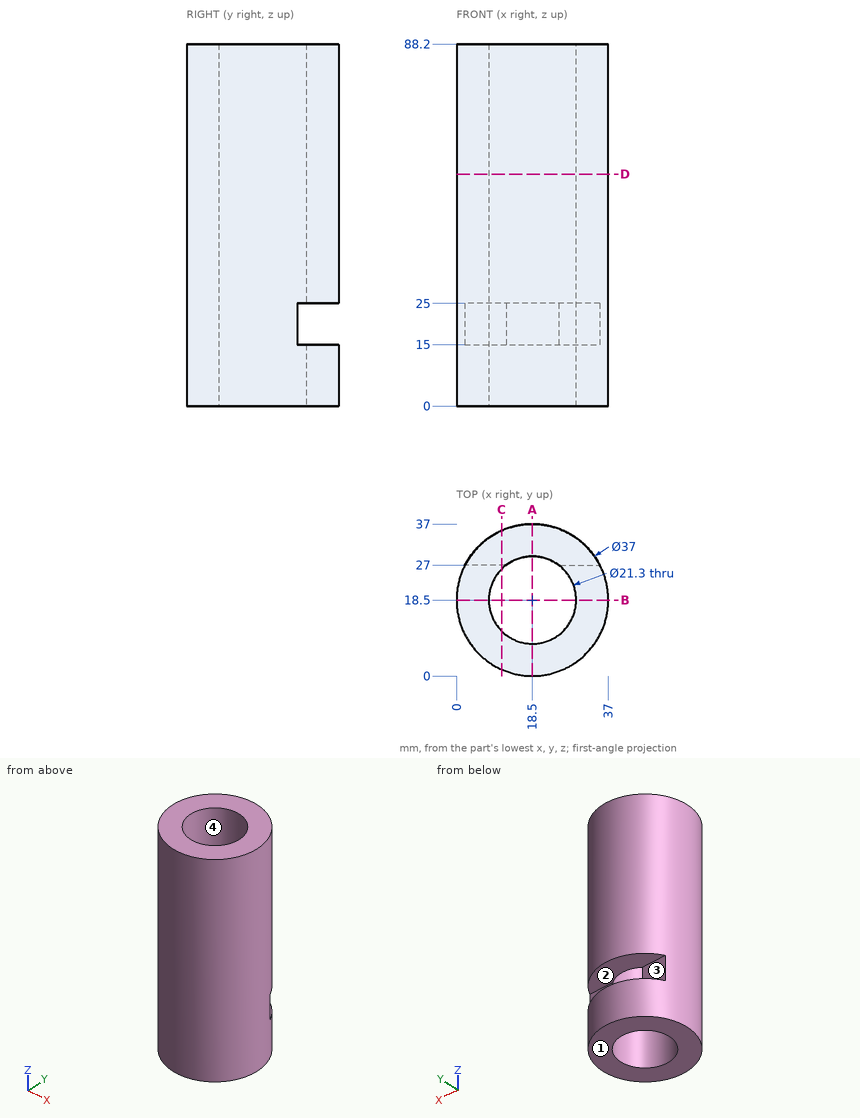
Answer from the drawing. Dimensions are ordinates in mm from the lowest x, y and z of the part. Give positions to 0.01 mm unless a question says otherwise; leave off trailing zeros. Order: outer loops, then holes, each group sorted by start corner. A loop starts at its lowest first (then second) coordinate and runs counter-clockwise, first axis right, second up.
Item 1: For a pull along Z with two mould halves and no side action, classify the marked faces 1, 2, 3 and 4 as pulls with the +Z half, pulls with the -Z half, needs draft (parallel to the pull), parting line crosses it, or undercut.
From the geometry:
face 1: pulls with the -Z half
face 2: undercut
face 3: undercut
face 4: needs draft
Item 2: The part is cut by section B-B, the plane y = 18.5. Give the vertices of the cut face in (x, z).
From the geometry:
outline: (0, 0) - (7.85, 0) - (7.85, 88.2) - (0, 88.2) - close; (29.15, 0) - (37, 0) - (37, 88.2) - (29.15, 88.2) - close
Item 3: The part is cut by section D-D, the plane z = 56.5. Give the vertices of the cut face in (x, y), and give its area (3 significant figures).
From the geometry:
outline: circle Ø37 at (18.5, 18.5); hole circle Ø21.3 at (18.5, 18.5)
area: 719 mm2
Item 4: Given pin 1 Ø2 at (y, z) = (22.5, 73) entering from +X; pin 2 Ø4 at (y, z) = (12.5, 32.5) entering from +X; pin 3 Ø4 at (x, z) = (11.5, 10) entering from -Y; pin 4 Ø4 at (x, y) = (21.5, 31) entering from -Z, each flat-ended and moving along its own axis, determine where each tip first touches the part or whether it passes through.
From the geometry:
pin 1: stops at x = 36.76
pin 2: stops at x = 36.56
pin 3: stops at y = 0.69
pin 4: stops at z = 0
Item 5: The part is cut by section C-C, the plane x = 11. Give the vertices of the cut face in (y, z).
From the geometry:
outline: (1.59, 0) - (10.94, 0) - (10.94, 88.2) - (1.59, 88.2) - close; (26.06, 0) - (35.41, 0) - (35.41, 15) - (27, 15) - (27, 25) - (35.41, 25) - (35.41, 88.2) - (26.06, 88.2) - close
Item 6: The part is cut by section A-A, the plane x = 18.5. Give the vertices of the cut face in (y, z), and give its area (3 significant figures).
From the geometry:
outline: (0, 0) - (7.85, 0) - (7.85, 88.2) - (0, 88.2) - close; (29.15, 0) - (37, 0) - (37, 15) - (29.15, 15) - close; (29.15, 25) - (37, 25) - (37, 88.2) - (29.15, 88.2) - close
area: 1,310 mm2
Item 7: Find the intervals of material crossed by probe 1 along Z at (x, y) = (29, 33); probe 2 along Y at (x, z) = (18.5, 55.5); probe 3 along X at (y, z) = (18, 33), in increasing order.
From the geometry:
probe 1: z = 0 to 15, 25 to 88.2
probe 2: y = 0 to 7.85, 29.15 to 37
probe 3: x = 0.01 to 7.86, 29.14 to 36.99
